Could you check a few things on this model? Use its own coordinates, in mm. A direction names the side the tool comes from. Round coordinates to 2 decimals unless told otherwise and drop trailing zeros. Loops run counter-clockwise (first coordinate to the right, second up) from the corner with the lowest first, then second, coordinate; pieces in that order, holes last. Notation, with made-up numbers: (82.25, 84) -> (95.25, 84) arc R26 ccw to (95.25, 101) -> close; hole circle Ø7 at (81.25, 62.25). An arc over 180 degrees is marked (long way). One line per item, written item: value.
```python
from build123d import *

# Parameters (mm, degrees)
SCHIZZO1_W                   = 45
SCHIZZO1_H                   = 20
ESTRUSIONE_ESTRUSIONE1_DEPTH = 3.1
SCHIZZO2_R                   = 8
ESTRUSIONE_ESTRUSIONE2_DEPTH = 13.5
SCHIZZO3_W                   = 7.5
SCHIZZO3_H                   = 3
ESTRUSIONE_ESTRUSIONE3_DEPTH = 4
ESTRUSIONE_ESTRUSIONE4_DEPTH = 3.5
SCHIZZO5_W                   = 7.5
SCHIZZO5_H                   = 2.5
ESTRUSIONE_ESTRUSIONE5_DEPTH = 7


with BuildPart() as part:
    # Schizzo1 → Estrusione-Estrusione1 (new body)
    with BuildSketch(Plane.XY):
        with Locations((22.5, 10)):
            Rectangle(SCHIZZO1_W, SCHIZZO1_H)
    extrude(amount=ESTRUSIONE_ESTRUSIONE1_DEPTH)

    # Schizzo2 → Estrusione-Estrusione2 (add)
    with BuildSketch(Plane.XY.offset(3.1)):
        with Locations(Location((9, 10, 0), (0, 0, 180))):
            Circle(SCHIZZO2_R)
        with Locations(Location((36, 10, 0), (0, 0, 180))):
            Circle(SCHIZZO2_R)
    extrude(amount=ESTRUSIONE_ESTRUSIONE2_DEPTH)

    # Schizzo3 → Estrusione-Estrusione3 (add)
    with BuildSketch(Plane(origin=(0, 0, 0), x_dir=(-1, 0, 0), z_dir=(0, 0, -1))):
        with Locations((-22.5, 1.5)):
            Rectangle(SCHIZZO3_W, SCHIZZO3_H)
    extrude(amount=ESTRUSIONE_ESTRUSIONE3_DEPTH)

    # Schizzo4 → Estrusione-Estrusione4 (add)
    with BuildSketch(Plane.XY.offset(3.1)):
        with BuildLine():
            Line((18.75, 20), (26.25, 20))
            ThreePointArc((26.25, 20), (28, 18.25), (26.25, 16.5))
            Line((26.25, 16.5), (18.75, 16.5))
            ThreePointArc((18.75, 16.5), (17, 18.25), (18.75, 20))
        make_face()
    extrude(amount=ESTRUSIONE_ESTRUSIONE4_DEPTH)

    # Schizzo5 → Estrusione-Estrusione5 (add)
    with BuildSketch(Plane.XZ):
        with Locations((22.5, -2.75)):
            Rectangle(SCHIZZO5_W, SCHIZZO5_H)
    extrude(amount=ESTRUSIONE_ESTRUSIONE5_DEPTH)


solid = part.part
```
(1) On a 3-axis mill with a long thin cutter (end or side, diameter ignored), from which of +Z, -Z, +X, -X, +Y, -Y can I reach the whole of each face in a straight line? I mean faces 4 (the face through (28, 18.3, 4.8)), 5 (the face through (22, -3, -1.5)), 6 (the face through (26.25, -2, -2)), 7 (the face through (23, 18, 6.6)). Say none if no direction works.
Results below:
face 4: +Z
face 5: +Z, +X, -X, -Y
face 6: -Z, +X, +Y, -Y
face 7: +Z, +Y, -Y
(2) We'd pull the mould along X, two halves only. Please class faces 1 (the face through (22, -7, -3)), 2 (the face through (23, 16.5, 5)), 3 (the face through (0, 10, 2)): +X half, -X half, draft (parallel to the pull), parting line (faces both ways), or undercut.
Results below:
face 1: draft
face 2: undercut
face 3: -X half
(3) Imagine slicing it at A-A on x = 36. Write out the boundary of the cut face in (y, z), then the cut area to 3 significant figures.
Results below:
outline: (0, 0) -> (20, 0) -> (20, 3.1) -> (18, 3.1) -> (18, 16.6) -> (2, 16.6) -> (2, 3.1) -> (0, 3.1) -> close
area: 278 mm²
(4) For pin 1 Ø10 at (y, z) = (-2, 10) entering from +X; pin 2 Ø12 at (y, z) = (-1, 11) entering from -X (3 decimals); pin 3 Ø1 at (x, z) = (31, 5.5) entering from +Y; pin 4 Ø4 at (y, z) = (-1.5, 11) entering from -X, each with a flat end and sliding along its axis, tell me the tip position at first contact or that it passes through.
Results below:
pin 1: stops at x = 39.87
pin 2: stops at x = 2.755
pin 3: stops at y = 16.61
pin 4: passes through
(5) Imagine slicing it at C-C on z = 12.75. Write out the boundary of the cut face in (x, y).
Results below:
outline: circle Ø16 at (9, 10); circle Ø16 at (36, 10)
(6) Imagine slicing it at D-D on y = 13. Write out the boundary of the cut face in (x, z), then the cut area to 3 significant figures.
Results below:
outline: (0, 0) -> (45, 0) -> (45, 3.1) -> (43.42, 3.1) -> (43.42, 16.6) -> (28.58, 16.6) -> (28.58, 3.1) -> (16.42, 3.1) -> (16.42, 16.6) -> (1.58, 16.6) -> (1.58, 3.1) -> (0, 3.1) -> close
area: 540 mm²
(7) Please list where these lines run through material, in increasing order: L1, parallel to Z at x = 5.5, y = 16; L2, parallel to Y at x = 26, z = 3.25; L3, parallel to Z at x = 42, y = 1.
Results below:
L1: z = 0 to 16.6
L2: y = 16.5 to 20
L3: z = 0 to 3.1
(8) Imagine slicing it at B-B on y = 10. Write out the boundary of the cut face in (x, z), then the cut area to 4 significant figures.
Results below:
outline: (0, 0) -> (45, 0) -> (45, 3.1) -> (44, 3.1) -> (44, 16.6) -> (28, 16.6) -> (28, 3.1) -> (17, 3.1) -> (17, 16.6) -> (1, 16.6) -> (1, 3.1) -> (0, 3.1) -> close
area: 571.5 mm²
